```python
from build123d import *

# Parameters (mm, degrees)
BOSS_EXTRU_1_DEPTH      = 5.08
ESQUISSE3_W             = 0.8
ESQUISSE3_H             = 1.27
ENL_V_MAT_EXTRU_1_DEPTH = 8.9
ESQUISSE4_W             = 2.4
ESQUISSE4_H             = 0.5
ENL_V_MAT_EXTRU_2_DEPTH = 6.08
ESQUISSE2_W             = 0.6
ESQUISSE2_H             = 0.6
BOSS_EXTRU_2_DEPTH      = 3.5
BOSS_EXTRU_2_DEPTH_BACK = 9
BOSS_EXTRU_3_DEPTH      = 2.54
CHANFREIN4_SIZE         = 0.15
CHANFREIN5_SIZE         = 0.4


with BuildPart() as part:
    # Esquisse1 → Boss.-Extru.1 (new body)
    with BuildSketch(Plane.XY):
        Polygon((0, 11.4), (0, 0), (5, 0), (5, 11.4), (4.2, 11.4), (4.2, 2.5), (0.8, 2.5), (0.8, 11.4), align=None)
    extrude(amount=BOSS_EXTRU_1_DEPTH)

    # Esquisse3 → Enlèv. mat.-Extru.1 (cut)
    with BuildSketch(Plane(origin=(0, 11.4, 0), x_dir=(1, 0, 0), z_dir=(0, 1, 0))):
        with Locations((0.4, -0.635)):
            Rectangle(ESQUISSE3_W, ESQUISSE3_H)
        with Locations((0.4, -4.445)):
            Rectangle(ESQUISSE3_W, ESQUISSE3_H)
    extrude(amount=-ENL_V_MAT_EXTRU_1_DEPTH, mode=Mode.SUBTRACT)

    # Esquisse4 → Enlèv. mat.-Extru.2 (cut, through all)
    with BuildSketch(Plane.XY.offset(5.08)):
        with Locations((2.5, 0.25)):
            Rectangle(ESQUISSE4_W, ESQUISSE4_H)
    extrude(amount=-ENL_V_MAT_EXTRU_2_DEPTH, mode=Mode.SUBTRACT)

    # Esquisse2 → Boss.-Extru.2 (add, two sides)
    with BuildSketch(Plane.XZ.offset(-0.5)) as boss_extru_2_sk:
        with Locations((2.5, 3.81)):
            Rectangle(ESQUISSE2_W, ESQUISSE2_H)
        with Locations((2.5, 1.27)):
            Rectangle(ESQUISSE2_W, ESQUISSE2_H)
    extrude(amount=BOSS_EXTRU_2_DEPTH)
    extrude(boss_extru_2_sk.sketch, amount=-BOSS_EXTRU_2_DEPTH_BACK)

    # Esquisse5 → Boss.-Extru.3 (add)
    with BuildSketch(Plane.XY.offset(3.81)):
        Polygon((0.8, 9.5), (1.2, 8.5), (0.8, 8.5), align=None)
    extrude(amount=-BOSS_EXTRU_3_DEPTH)

    # Chanfrein4
    chanfrein4_edges = [part.edges().sort_by_distance(p)[0] for p in [
        (2.8, 9.5, 3.81),
        (2.5, 9.5, 3.51),
        (2.2, 9.5, 3.81),
        (2.5, 9.5, 4.11),
        (2.8, -3, 3.81),
        (2.5, -3, 4.11),
        (2.2, -3, 3.81),
        (2.5, -3, 3.51),
        (2.8, 9.5, 1.27),
        (2.5, 9.5, 0.97),
        (2.2, 9.5, 1.27),
        (2.5, 9.5, 1.57),
        (2.8, -3, 1.27),
        (2.5, -3, 1.57),
        (2.2, -3, 1.27),
        (2.5, -3, 0.97),
    ]]
    chamfer(chanfrein4_edges, length=CHANFREIN4_SIZE)

    # Chanfrein5
    chanfrein5_edges = [part.edges().sort_by_distance(p)[0] for p in [
        (4.2, 11.4, 2.54),
        (0.8, 11.4, 2.54),
    ]]
    chamfer(chanfrein5_edges, length=CHANFREIN5_SIZE)


solid = part.part
```
The listing builds one solid part. Answer for the finished solid, in the listing's coordinates (mm). A direction names the side the tool comes from. Give positions to 0.01 mm unless a question says otherwise; leave off trailing zeros. Order: outer loops, then holes, each group sorted by start corner. A loop starts at its lowest first (then second) coordinate and runs counter-clockwise, first axis right, second up. Notation, with made-up numbers: (-19, 34) -> (-13, 34) arc R20 cw to (-13, 45) -> close; hole circle Ø8 at (-36.75, 10.25). An arc over 180 degrees is marked (long way). Answer as CSV lines item,"result". Start each with the question number.
Q1. Determine the mould class of faces 5 (the flat face through (2, 2.5, 3)), 6 (the flat face through (2, 0.5, 3)), 7 (the flat face through (0, 5, 3)), 8 (the flat face through (4, 0, 3)) for opening direction X: pulls with the +X half, pulls with the -X half, needs draft (parallel to the pull), parting line crosses it, or undercut.
Q2. Given pin 1 (0.5 mm diameter, centred on x = 2.5, y = -0.5, fed in from +Z); pin 2 (0.7 mm diameter, centred on y = -1.5, z = 1.5, fed in from -X); pin 3 (3 mm diameter, centred on x = 2.5, y = 8.5, fed in from -Z), each flat-ended and moving along its own axis, determine where each tip first touches the part or whether it passes through.
Q3. A cutting plane is placed at B-B (x = 0.55). Determine the outline of the cut face in (y, z), then the cut area to 3 significant figures.
Q4. Find the intervals of material crossed by L1, parallel to X at y = 6.25, z = 3.65; L2, parallel to X at y = 4.5, z = 1.2; L3, parallel to X at y = 4.25, z = 1.6, in increasing order.
Q5. A cutting plane is placed at A-A (y = 5.5). Determine the outline of the cut face in (x, z), then the cut area to 3 significant figures.
Q6. A cutting plane is placed at C-C (y = -2). Determine the outline of the cut face in (x, z).
Q7. A cutting plane is placed at D-D (z = 3.35). Determine the outline of the cut face in (x, y), then the cut area to 3 significant figures.
Q8. Which of the six approach directions +Z, -Z, +X, -X, +Y, -Y give full straight-line access (tool end or side, diameter ignored) to faces 1 (the flat face through (0.8, 5, 3)), 2 (the flat face through (0.5, 7, 1.27)), 3 (the flat face through (1, 0, 3)), 4 (the flat face through (0.8, 10, 3))?
Results found:
1,face 5,"undercut"
1,face 6,"undercut"
1,face 7,"pulls with the -X half"
1,face 8,"needs draft"
2,pin 1,"z = 4.11"
2,pin 2,"x = 2.2"
2,pin 3,"z = 0.97"
3,outline,"(0, 0) -> (2.5, 0) -> (2.5, 1.27) -> (11.25, 1.27) -> (11.25, 3.81) -> (2.5, 3.81) -> (2.5, 5.08) -> (0, 5.08) -> close"
3,area,"34.9 mm2"
4,L1,"0 to 0.8, 2.2 to 2.8, 4.2 to 5"
4,L2,"2.2 to 2.8, 4.2 to 5"
4,L3,"0 to 0.8, 4.2 to 5"
5,outline,"(0, 1.27) -> (0.8, 1.27) -> (0.8, 3.81) -> (0, 3.81) -> close; (2.2, 0.97) -> (2.8, 0.97) -> (2.8, 1.57) -> (2.2, 1.57) -> close; (2.2, 3.51) -> (2.8, 3.51) -> (2.8, 4.11) -> (2.2, 4.11) -> close; (4.2, 0) -> (5, 0) -> (5, 5.08) -> (4.2, 5.08) -> close"
5,area,"6.82 mm2"
6,outline,"(2.2, 0.97) -> (2.8, 0.97) -> (2.8, 1.57) -> (2.2, 1.57) -> close; (2.2, 3.51) -> (2.8, 3.51) -> (2.8, 4.11) -> (2.2, 4.11) -> close"
7,outline,"(0, 0) -> (1.3, 0) -> (1.3, 0.5) -> (3.7, 0.5) -> (3.7, 0) -> (5, 0) -> (5, 11.4) -> (4.6, 11.4) -> (4.2, 11) -> (4.2, 2.5) -> (0.8, 2.5) -> (0.8, 8.5) -> (1.2, 8.5) -> (0.8, 9.5) -> (0.8, 11) -> (0.4, 11.4) -> (0, 11.4) -> close"
7,area,"25.6 mm2"
8,face 1,"+Z, -Z"
8,face 2,"-Z, -X, +Y"
8,face 3,"+Z, -Z, -X, -Y"
8,face 4,"+Z, -Z, +Y"
